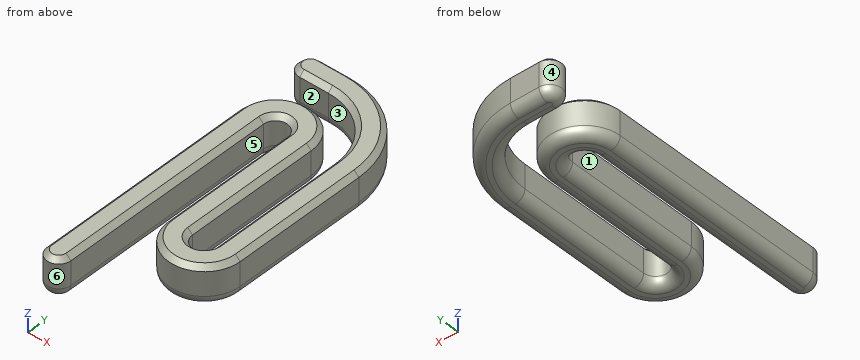
from build123d import *

# Parameters (mm, degrees)
F1_DEPTH = 8
F2_R     = 2
F3_SIZE  = 1


with BuildPart() as f1:
    # F0 (on Top) → F1 (new body)
    with BuildSketch(Plane.XY):
        with BuildLine():
            ThreePointArc((-20.181158, -13.582748), (-18.804883, -9.252621), (-15.181158, -6.51168))
            Line((-15.181158, -6.51168), (-15.181158, 14.463018))
            ThreePointArc((-15.181158, 14.463018), (-22.681158, 21.963018), (-30.181158, 14.463018))
            Line((-30.181158, 14.463018), (-30.181158, -16.082748))
            Line((-30.181158, -16.082748), (-30.181158, -31.082748))
            ThreePointArc((-30.181158, -31.082748), (-27.681158, -33.582748), (-25.181158, -31.082748))
            Line((-25.181158, -31.082748), (-25.181158, -16.082748))
            Line((-25.181158, -16.082748), (-25.181158, 14.463018))
            ThreePointArc((-25.181158, 14.463018), (-22.681158, 16.963018), (-20.181158, 14.463018))
            Line((-20.181158, 14.463018), (-20.181158, -13.582748))
        make_face()
        with BuildLine():
            Line((-10.181158, 14.463018), (-10.181158, -6.51168))
            ThreePointArc((-10.181158, -6.51168), (-6.557434, -9.252621), (-5.181158, -13.582748))
            Line((-5.181158, -13.582748), (-5.181158, 14.463018))
            ThreePointArc((-5.181158, 14.463018), (-10.306789, 26.837386), (-22.681158, 31.963018))
            Line((-22.681158, 31.963018), (-28.681158, 31.963018))
            ThreePointArc((-28.681158, 31.963018), (-31.181158, 29.463018), (-28.681158, 26.963018))
            Line((-28.681158, 26.963018), (-22.681158, 26.963018))
            ThreePointArc((-22.681158, 26.963018), (-13.842323, 23.301852), (-10.181158, 14.463018))
        make_face()
        with BuildLine():
            ThreePointArc((-10.181158, -13.582748), (-12.681158, -16.082748), (-15.181158, -13.582748))
            Line((-15.181158, -13.582748), (-15.181158, -6.51168))
            ThreePointArc((-15.181158, -6.51168), (-18.804883, -9.252621), (-20.181158, -13.582748))
            ThreePointArc((-20.181158, -13.582748), (-12.681158, -21.082748), (-5.181158, -13.582748))
            ThreePointArc((-5.181158, -13.582748), (-6.557434, -9.252621), (-10.181158, -6.51168))
            Line((-10.181158, -6.51168), (-10.181158, -13.582748))
        make_face()
    extrude(amount=F1_DEPTH)

    # F2
    f2_edges = [f1.edges().sort_by_distance(p)[0] for p in [
        (-5.181158, 0.440135, 0),
    ]]
    fillet(f2_edges, radius=F2_R)

    # F3
    f3_edges = [f1.edges().sort_by_distance(p)[0] for p in [
        (-20.181158, 0.440135, 8),
    ]]
    chamfer(f3_edges, length=F3_SIZE)


solid = f1.part
Read the model definition and answer for the solid it produces. Units are mm, in the model's axes. Face numbers are marked on the shaded views. A direction names the side the tool comes from. Round coordinates to 2 decimals unless told otherwise and drop trailing zeros. Write each loop counter-clockwise with the first axis right and the second up, starting at its lowest first coordinate (ties: lowest second). Pieces come first, ordered by that corner, then holes.
1. Given pin 1 Ø2 at (x, z) = (-8, 7) entering from +Y; pin 2 Ø2.5 at (y, z) = (-3, 4.5) entering from -X; pin 3 Ø1 at (x, z) = (-9, 1.5) entering from +Y, each flat-ended and moving along its own axis, determine where each tip first touches the part or whether it passes through.
2. The part is cut by section B-B, the plane z = 3.5. Determine the outline of the cut face in (x, y), then the cut area to 3 significant figures.
3. Determine the mould class of the marked faces 4, 5 and 6 for opening direction X: pulls with the +X half, pulls with the -X half, needs draft (parallel to the pull), parting line crosses it, or undercut.
4. Straight lines are drawn through the part: L1, parallel to X at y = 8.5, z = 5.75; L2, parallel to X at y = 10, z = 7.25; L3, parallel to Y at x = -12.25, z = 3. For each, find the intervals that lie inside material, in ascending order.
5. The part is cut by section C-C, the plane y = -25. Determine the outline of the cut face in (x, z).
6. The part is cut by section A-A, the plane y = -10. Determine the outline of the cut face in (x, z), then the cut area to 3 significant figures.
7. Which of the six approach directions +Z, -Z, +X, -X, +Y, -Y give full straight-line access (tool end or side, diameter ignored) to the marked faces 1, 2 and 3?
Values:
1. pin 1: stops at y = 25.38
1. pin 2: stops at x = -30.18
1. pin 3: stops at y = 25.9
2. outline: (-30.18, -31.08) arc R2.5 ccw to (-25.18, -31.08) - (-25.18, 14.46) arc R2.5 cw to (-20.18, 14.46) - (-20.18, -13.58) arc R7.5 ccw to (-5.18, -13.58) - (-5.18, 14.46) arc R17.5 ccw to (-22.68, 31.96) - (-28.68, 31.96) arc R2.5 ccw to (-28.68, 26.96) - (-22.68, 26.96) arc R12.5 cw to (-10.18, 14.46) - (-10.18, -13.58) arc R2.5 cw to (-15.18, -13.58) - (-15.18, 14.46) arc R7.5 ccw to (-30.18, 14.46) - close
2. area: 833 mm2
3. face 4: pulls with the -X half
3. face 5: undercut
3. face 6: parting line crosses it
4. L1: x = -30.18 to -25.18, -20.18 to -15.18, -10.18 to -5.18
4. L2: x = -29.93 to -25.43, -19.93 to -15.43, -9.93 to -5.43
4. L3: y = -21.07 to -16.05, 21.35 to 28.51
5. outline: (-30.18, 2) arc R2 ccw to (-28.18, 0) - (-27.18, 0) arc R2 ccw to (-25.18, 2) - (-25.18, 7) - (-26.18, 8) - (-29.18, 8) - (-30.18, 7) - close
6. outline: (-30.18, 2) arc R2 ccw to (-28.18, 0) - (-27.18, 0) arc R2 ccw to (-25.18, 2) - (-25.18, 7) - (-26.18, 8) - (-29.18, 8) - (-30.18, 7) - close; (-20.18, 2) arc R2 ccw to (-18.18, 0) - (-17.18, 0) arc R2 ccw to (-15.18, 2) - (-15.18, 7) - (-16.18, 8) - (-19.18, 8) - (-20.18, 7) - close; (-10.18, 2) arc R2 ccw to (-8.18, 0) - (-7.18, 0) arc R2 ccw to (-5.18, 2) - (-5.18, 7) - (-6.18, 8) - (-9.18, 8) - (-10.18, 7) - close
6. area: 112 mm2
7. face 1: +Z, -Z, -Y
7. face 2: +Z, -Z, -X
7. face 3: +Z, -Z
